from build123d import *

# Parameters (mm, degrees)
SKETCH2_R           = 5
SKETCH2_R_2         = 4
BOSS_EXTRUDE1_DEPTH = 10


with BuildPart() as part:
    # Sketch2 → Boss-Extrude1 (new body)
    with BuildSketch(Plane.XY):
        with BuildLine():
            Line((-125, 140), (125, 140))
            ThreePointArc((125, 140), (135.606601718, 135.606601718), (140, 125))
            Line((140, 125), (140, -125))
            ThreePointArc((140, -125), (135.606601718, -135.606601718), (125, -140))
            Line((125, -140), (-125, -140))
            ThreePointArc((-125, -140), (-135.606601718, -135.606601718), (-140, -125))
            Line((-140, -125), (-140, 125))
            ThreePointArc((-140, 125), (-135.606601718, 135.606601718), (-125, 140))
        make_face()
        with Locations((-125, 125)):
            Circle(SKETCH2_R, mode=Mode.SUBTRACT)
        with Locations((0, 125)):
            Circle(SKETCH2_R, mode=Mode.SUBTRACT)
        with Locations((125, 125)):
            Circle(SKETCH2_R, mode=Mode.SUBTRACT)
        Circle(SKETCH2_R_2, mode=Mode.SUBTRACT)
        with Locations((125, 0)):
            Circle(SKETCH2_R, mode=Mode.SUBTRACT)
        with Locations((-125, 0)):
            Circle(SKETCH2_R, mode=Mode.SUBTRACT)
        with Locations((-125, -125)):
            Circle(SKETCH2_R, mode=Mode.SUBTRACT)
        with Locations((0, -125)):
            Circle(SKETCH2_R, mode=Mode.SUBTRACT)
        with Locations((125, -125)):
            Circle(SKETCH2_R, mode=Mode.SUBTRACT)
    extrude(amount=BOSS_EXTRUDE1_DEPTH)


solid = part.part
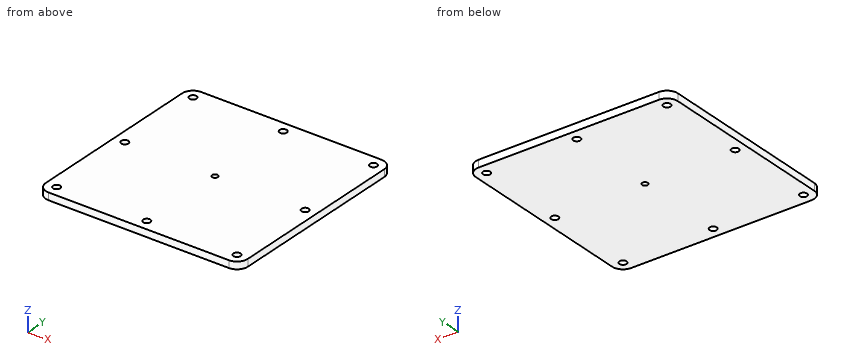
The listing builds one solid part. Answer for the finished solid, in the listing's coordinates (mm). Coordinates: 2 decimals unless noted, no trailing zeros. Write each loop counter-clockwise with the first axis right and the second up, starting at its lowest first coordinate (ties: lowest second). Pieces come first, ordered by that corner, then holes. Notation, with made-up numbers: (38.5, 77.25) - (82.5, 77.25) arc R9 cw to (82.5, 93.25) - close; hole circle Ø6 at (6.25, 31). An arc over 180 degrees is marked (long way). Return JSON: item names as keys, results as strings.
1. Consider line 1 along Y through (x, z) = (125, 7); line 2 along X through (y, z) = (-124, 8.25); line 3 along X through (y, z) = (121, 8.25). Determine where each line is inside the solid, lowest interval first.
Final values:
{"line 1": "-140 to -130, -120 to -5, 5 to 120, 130 to 140", "line 2": "-140 to -129.9, -120.1 to -4.9, 4.9 to 120.1, 129.9 to 140", "line 3": "-140 to -128, -122 to -3, 3 to 122, 128 to 140"}
2. The part is cut by section A-A on x = 0. Determine the outline of the cut face in (y, z), then the cut area to 3 significant figures.
Final values:
{"outline": "(-140, 0) - (-130, 0) - (-130, 10) - (-140, 10) - close; (-120, 0) - (-4, 0) - (-4, 10) - (-120, 10) - close; (4, 0) - (120, 0) - (120, 10) - (4, 10) - close; (130, 0) - (140, 0) - (140, 10) - (130, 10) - close", "area": "2,520 mm^2"}
